Model file for the job. Use its own axes, mm. A direction names the side the tool comes from. Round coordinates to 2 decimals unless told otherwise and drop trailing zeros. Order: outer loops, then holes, each group sorted by start corner. A loop starts at its lowest first (then second) coordinate and runs counter-clockwise, first axis right, second up. Notation, with made-up numbers: (14, 83) - (44, 83) arc R9 cw to (44, 96) - close; hole circle Ø5 at (16.25, 50). An arc over 180 degrees is marked (long way). Put each result on its own line as item: value. Start each with the question number.
Item 1: Saw through at B-B on x = -39.5. List the corners of the cut face in (y, z), plus the area to 3 significant figures.
Item 2: Probe probe 1 along Y at (x, z) = (-48, 47.5); probe 2 along Y at (x, z) = (-63.5, 25.5); probe 3 along X at (y, z) = (29.5, 56.5). List the from-to ranges inside material, lowest first.
Item 3: Pin check, flat tips, straight feed: pin 1 Ø1 at (y, z) = (79.5, 33.5) entering from -X; pin 2 Ø6 at (y, z) = (14, 58.5) entering from +X; pin 3 Ø1.5 at (y, z) = (2.5, 44) entering from +X. Stop position of each tip, or through.
Item 4: Mould opens along X. For faces 1 (the face through (-81.603, 24.714, 37.567)), 2 (the face through (-43, 0, 39)), 3 (the face through (-11.9, 30.5, 38.6)), 4 (the face through (-37, 5.08, 38)) say: pulls with the +X half, pulls with the -X half, needs draft (parallel to the pull), parting line crosses it, or undercut.
Item 5: Saw through at A-A on z = 63. List the corners of the cut face in (x, y).
Item 6: Saw through at D-D on x = -20. List the corners of the cut face in (y, z).
Item 7: Saw through at C-C on y = 39. List the corners of the cut face in (x, z), plus the area to 3 significant figures.
Item 8: Which spindle directions (+Z, -Z, +X, -X, +Y, -Y) get a long thin tool onto all of the face, cutting with end or side? Do faces 5 (the face through (-5, 80.3, 37.6)), 6 (the face through (-42, 4.08, 41)), 7 (the face through (-78.945, 9.097, 37.567)). Say none if no direction does.
```python
from build123d import *

# Parameters (mm, degrees)
F1_DEPTH    = 76.2
F2_W        = 76.2
F2_H        = 3.08
F3_DEPTH    = 71.12
F4_W        = 76.2
F4_H        = 2.54
F5_DEPTH    = 2.032
F6_T4_DEPTH = 76.2
F8_DEPTH    = 76.2


# Not quite as in the source:
# - a fillet or chamfer that OpenCascade refuses, or shapes differently, is made with other operations: its cross-section is extruded or revolved along the edge and cut away or added


with BuildPart() as f1:
    # F0 (on Top) → F1 (new body)
    with BuildSketch(Plane.XY):
        with BuildLine():
            Line((-71.12, 0), (-2.54, 0))
            ThreePointArc((-2.54, 0), (-0.7439487758, 0.7439487758), (0, 2.54))
            ThreePointArc((0, 2.54), (-0.7439487758, 4.3360512242), (-2.54, 5.08))
            Line((-2.54, 5.08), (-69.676465438, 5.08))
            ThreePointArc((-69.676465438, 5.08), (-79.0448551931, 9.2054286756), (-82.3268475088, 18.9015317486))
            ThreePointArc((-82.3268475088, 18.9015317486), (-78.2116767293, 22.3014792843), (-72.9571412523, 21.3611970334))
            Line((-72.9571412523, 21.3611970334), (-70.7962627974, 19.8481336501))
            Line((-70.7962627974, 19.8481336501), (-55.0490144099, 8.8217916231))
            Line((-55.0490144099, 8.8217916231), (11.9676564134, 104.5315164778))
            Line((11.9676564134, 104.5315164778), (9.8870102209, 105.9884006261))
            Line((9.8870102209, 105.9884006261), (-55.672776454, 12.3593219639))
            Line((-55.672776454, 12.3593219639), (-71.2776228977, 23.2859530764))
            ThreePointArc((-71.2776228977, 23.2859530764), (-81.747690686, 24.661984001), (-88.8767730732, 16.871479209))
            Line((-88.8767730732, 16.871479209), (-88.8912459344, 6.3587420222))
            ThreePointArc((-88.8912459344, 6.3587420222), (-87.0344697211, 1.8629637755), (-82.541251952, 0))
            Line((-82.541251952, 0), (-71.12, 0))
        make_face()
    extrude(amount=F1_DEPTH)

    # F2 (on face) → F3 (cut)
    with BuildSketch(Plane.XY.offset(76.2)):
        with Locations((-41.91, 2.54)):
            Rectangle(F2_W, F2_H)
    extrude(amount=-F3_DEPTH, mode=Mode.SUBTRACT)

    # F4 (on Front) → F5 (join)
    with BuildSketch(Plane.XZ):
        with Locations((-41.91, 74.93)):
            Rectangle(F4_W, F4_H)
    extrude(amount=-F5_DEPTH)

    # F6: chamfer of 2.54 on 1 edges, made by hand


with BuildPart() as f6_tool2:
    # F6_s3 → F6_t4 (new body)
    with BuildSketch(Plane.YZ.offset(-80.01)):
        Polygon((-0.508, 73.66), (2.032, 76.2), (2.032, 73.66), align=None)
    extrude(amount=F6_T4_DEPTH)

    split(bisect_by=Plane.XZ.offset(-1), keep=Keep.BOTTOM)


with BuildPart() as f1_1:
    add(f1.part)

    # F6_t1: cut F6_tool2
    add(f6_tool2.part, mode=Mode.SUBTRACT)

    # F7 (on face) → F8 (join)
    with BuildSketch(Plane.XY.offset(76.2)):
        Polygon((-4.6713010828, 5.08), (-2.54, 5.08), (-21.5406789982, 56.6766540504), (-22.9374096266, 54.6819159876), align=None)
    extrude(amount=-F8_DEPTH)


solid = f1_1.part
```
Results found:
1. outline: (0, 0) - (5.08, 0) - (5.08, 76.2) - (4.08, 76.2) - (4.08, 5.08) - (1, 5.08) - (1, 75.17) - (2.03, 76.2) - (0, 76.2) - close; (31.03, 0) - (35.46, 0) - (35.46, 76.2) - (31.03, 76.2) - close
1. area: 506 mm²
2. probe 1: y = 0 to 1, 4.08 to 5.08, 18.89 to 23.32
2. probe 2: y = 0 to 1, 4.08 to 5.08, 14.74 to 17.84
2. probe 3: x = -43.67 to -40.57, -13.66 to -11.53
3. pin 1: stops at x = -9.01
3. pin 2: stops at x = -4.72
3. pin 3: stops at x = 0
4. face 1: undercut
4. face 2: needs draft
4. face 3: pulls with the +X half
4. face 4: undercut
5. outline: (-88.89, 6.36) arc R6.35 ccw to (-82.54, 0) - (-2.54, 0) arc R2.54 ccw to (-2.54, 5.08) - (-21.54, 56.68) - (11.97, 104.53) - (9.89, 105.99) - (-55.67, 12.36) - (-71.28, 23.29) arc R11.43 ccw to (-88.88, 16.87) - close; hole (-82.33, 18.9) arc R12.7 ccw to (-69.68, 5.08) - (-4.67, 5.08) - (-22.94, 54.68) - (-55.05, 8.82) - (-72.96, 21.36) arc R6.35 ccw to start; hole (-80.01, 1) - (-3.81, 1) - (-3.81, 4.08) - (-80.01, 4.08) - close
6. outline: (0, 0) - (5.08, 0) - (5.08, 76.2) - (4.08, 76.2) - (4.08, 5.08) - (1, 5.08) - (1, 75.17) - (2.03, 76.2) - (0, 76.2) - close; (46.71, 0) - (52.49, 0) - (52.49, 76.2) - (46.71, 76.2) - close; (58.88, 0) - (63.31, 0) - (63.31, 76.2) - (58.88, 76.2) - close
7. outline: (-37.02, 0) - (-33.92, 0) - (-33.92, 76.2) - (-37.02, 76.2) - close; (-17.16, 0) - (-15.03, 0) - (-15.03, 76.2) - (-17.16, 76.2) - close
7. area: 399 mm²
8. face 5: +Z, -Z, +X
8. face 6: +Z
8. face 7: +Z, -Z
